```python
from build123d import *

# Parameters (mm, degrees)
F1_W     = 28
F1_H     = 580
F3_DEPTH = 60
F2_W     = 40
F2_H     = 60
F4_DEPTH = 60


with BuildPart() as f3:
    # F1 (on face) → F3 (new body)
    with BuildSketch(Plane.XY):
        Polygon((1037.666667, 1779.203768), (-1518.333333, 1779.203768), (-1518.333333, 1419.203768), (-1518.333333, 1143.203768), (1037.666667, 1143.203768), align=None)
        Polygon((-1490.333333, 1171.203768), (-1490.333333, 1751.203768), (-990.333333, 1751.203768), (-962.333333, 1751.203768), (-518.333333, 1751.203768), (-490.333333, 1751.203768), (-18.333333, 1751.203768), (9.666667, 1751.203768), (481.666667, 1751.203768), (509.666667, 1751.203768), (1009.666667, 1751.203768), (1009.666667, 1171.203768), (509.666667, 1171.203768), (481.666667, 1171.203768), (9.666667, 1171.203768), (-18.333333, 1171.203768), (-490.333333, 1171.203768), (-518.333333, 1171.203768), (-962.333333, 1171.203768), (-990.333333, 1171.203768), align=None, mode=Mode.SUBTRACT)
        with Locations((-976.333333, 1461.203768)):
            Rectangle(F1_W, F1_H)
        with Locations((-504.333333, 1461.203768)):
            Rectangle(F1_W, F1_H)
        with Locations((-4.333333, 1461.203768)):
            Rectangle(F1_W, F1_H)
        with Locations((495.666667, 1461.203768)):
            Rectangle(F1_W, F1_H)
    extrude(amount=F3_DEPTH)

    # F2 (on face) → F4 (join)
    with BuildSketch(Plane.XY):
        with Locations((-1470.333333, 1721.203768)):
            Rectangle(F2_W, F2_H)
    extrude(amount=F4_DEPTH)


solid = f3.part
```
Check sheet for the modelled part. Datum: model origin and axes. Units: mm. A direction names the side the tool comes from. Round coordinates to 2 decimals unless told otherwise and drop trailing zeros. Write each loop counter-clockwise with the first axis right and the second up, starting at its lowest first coordinate (ties: lowest second). Pieces come first, ordered by that corner, then holes. Notation, with made-up numbers: (-35, 42) -> (-23, 42) arc R23 ccw to (-23, 64) -> close; hole circle Ø10 at (16.5, 36.5). An arc over 180 degrees is marked (long way). Put each result on its own line as item: value.
(1) Sectioned sample at B-B (z = 40). Enter the section's corners in (x, y).
Values found:
outline: (-1518.33, 1143.2) -> (1037.67, 1143.2) -> (1037.67, 1779.2) -> (-1518.33, 1779.2) -> close; hole (-1490.33, 1171.2) -> (-990.33, 1171.2) -> (-990.33, 1751.2) -> (-1450.33, 1751.2) -> (-1450.33, 1691.2) -> (-1490.33, 1691.2) -> close; hole (-962.33, 1171.2) -> (-518.33, 1171.2) -> (-518.33, 1751.2) -> (-962.33, 1751.2) -> close; hole (-490.33, 1171.2) -> (-18.33, 1171.2) -> (-18.33, 1751.2) -> (-490.33, 1751.2) -> close; hole (9.67, 1171.2) -> (481.67, 1171.2) -> (481.67, 1751.2) -> (9.67, 1751.2) -> close; hole (509.67, 1171.2) -> (1009.67, 1171.2) -> (1009.67, 1751.2) -> (509.67, 1751.2) -> close
(2) Material ranges on line 1 (X direction, y = 1667.5, z = 9.5); line 2 (X direction, y = 1741, z = 16.5); line 3 (Y direction, x = 281.5, z = 42.5), recorded low to high.
Values found:
line 1: x = -1518.33 to -1490.33, -990.33 to -962.33, -518.33 to -490.33, -18.33 to 9.67, 481.67 to 509.67, 1009.67 to 1037.67
line 2: x = -1518.33 to -1450.33, -990.33 to -962.33, -518.33 to -490.33, -18.33 to 9.67, 481.67 to 509.67, 1009.67 to 1037.67
line 3: y = 1143.2 to 1171.2, 1751.2 to 1779.2
(3) Sectioned sample at C-C (x = -1275.5). Enter the section's corners in (y, z).
Values found:
outline: (1143.2, 0) -> (1171.2, 0) -> (1171.2, 60) -> (1143.2, 60) -> close; (1751.2, 0) -> (1779.2, 0) -> (1779.2, 60) -> (1751.2, 60) -> close
(4) Sectioned sample at A-A (y = 1658). Enter the section's corners in (x, z), plus the area to 3 significant figures.
Values found:
outline: (-1518.33, 0) -> (-1490.33, 0) -> (-1490.33, 60) -> (-1518.33, 60) -> close; (-990.33, 0) -> (-962.33, 0) -> (-962.33, 60) -> (-990.33, 60) -> close; (-518.33, 0) -> (-490.33, 0) -> (-490.33, 60) -> (-518.33, 60) -> close; (-18.33, 0) -> (9.67, 0) -> (9.67, 60) -> (-18.33, 60) -> close; (481.67, 0) -> (509.67, 0) -> (509.67, 60) -> (481.67, 60) -> close; (1009.67, 0) -> (1037.67, 0) -> (1037.67, 60) -> (1009.67, 60) -> close
area: 10,100 mm^2
(5) Mould release check, pull along X, two halves, no side actions. Record for faces 3 (the face through (-341, 1769, 0)), 4 (the face through (756, 1751.204, 30)), 5 (the face through (-1518.333, 1466, 30)): released by +X, released by -X, zero draft, split by the parting line, or undercut.
Values found:
face 3: zero draft
face 4: undercut
face 5: released by -X
(6) Tool access check on faces 1 (the face through (481.667, 1457, 30)), 2 (the face through (1037.667, 1457, 30)). Record the directions out of +Z, -Z, +X, -X, +Y, -Y that give a thin tool (end or side, any length) a straight path to the whole face; none if there is none.
Values found:
face 1: +Z, -Z
face 2: +Z, -Z, +X, +Y, -Y
